Verification items for the finished model (mm, model axes). A direction names the side the tool comes from. Round coordinates to 2 decimals unless told otherwise and drop trailing zeros. Write each loop counter-clockwise with the first axis right and the second up, starting at its lowest first coordinate (ties: lowest second). Pieces come first, ordered by that corner, then holes. Notation, with made-up numbers: M 60,6 L 101,6 A16 ccw 101,23 Z; hole C -14.5,21.25 d7. An arc over 180 degrees is marked long. One line per item, written item: value. Start each with the question number.
from build123d import *

# Parameters (mm, degrees)
F0_R      = 146.05
F1_DEPTH  = 63.5
F2_R      = 142.875
F3_DEPTH  = 57.15
F5_DEPTH  = 57.15
F7_DEPTH  = 63.501
F8_W      = 381
F8_H      = 63.5
F9_DEPTH  = 6.35
F10_W     = 19.7993
F10_H     = 39.899997
F11_DEPTH = 6.35
F12_W     = 19.89836
F12_H     = 39.878
F13_DEPTH = 6.35
F14_R     = 50.8
F15_DEPTH = 6.35
F16_W     = 101.6
F16_H     = 81.28
F17_DEPTH = 63.501


with BuildPart() as f1:
    # F0 (on Top) → F1 (new body)
    with BuildSketch(Plane.XY):
        Circle(F0_R)
    extrude(amount=F1_DEPTH)

    # F2 (on face) → F3 (cut)
    with BuildSketch(Plane.XY.offset(63.5)):
        Circle(F2_R)
    extrude(amount=-F3_DEPTH, mode=Mode.SUBTRACT)

    # F4 (on face) → F5 (cut)
    with BuildSketch(Plane.XY.offset(63.5)):
        with BuildLine():
            Line((142.875, 0), (186.450183, 0))
            Line((186.450183, 0), (186.450183, 147.836223))
            Line((186.450183, 147.836223), (-190.863192, 147.836223))
            Line((-190.863192, 147.836223), (-190.863192, 0))
            Line((-190.863192, 0), (-142.875, 0))
            ThreePointArc((-142.875, 0), (0, 142.875), (142.875, 0))
        make_face()
    extrude(amount=-F5_DEPTH, mode=Mode.SUBTRACT)

    # F6 (on face) → F7 (cut, through all)
    with BuildSketch(Plane.XY.offset(63.5)):
        with BuildLine():
            Line((0, 0), (94.561977, 127.513117))
            ThreePointArc((94.561977, 127.513117), (0, 159.458628), (-94.561977, 127.513117))
            Line((-94.561977, 127.513117), (0, 0))
        make_face()
    extrude(amount=-F7_DEPTH, mode=Mode.SUBTRACT)

    # F8 (on Top) → F9 (join)
    with BuildSketch(Plane.XY):
        with Locations((0, 0.073786)):
            Rectangle(F8_W, F8_H)
    extrude(amount=F9_DEPTH)

    # F10 (on face) → F11 (cut)
    with BuildSketch(Plane.XY.offset(6.35)):
        with Locations((-159.01035, -0.826213)):
            Rectangle(F10_W, F10_H)
    extrude(amount=-F11_DEPTH, mode=Mode.SUBTRACT)

    # F12 (on Top) → F13 (cut)
    with BuildSketch(Plane.XY):
        with Locations((158.96082, -0.815214)):
            Rectangle(F12_W, F12_H)
    extrude(amount=F13_DEPTH, mode=Mode.SUBTRACT)

    # F14 (on Top) → F15 (cut)
    with BuildSketch(Plane.XY):
        Circle(F14_R)
    extrude(amount=F15_DEPTH, mode=Mode.SUBTRACT)

    # F16 (on Top) → F17 (cut, through all)
    with BuildSketch(Plane.XY):
        with Locations((0, 40.64)):
            Rectangle(F16_W, F16_H)
    extrude(amount=F17_DEPTH, mode=Mode.SUBTRACT)


solid = f1.part
1) Cross-section at B-B (z = 40). Record the boundary of the cut face in (x, y) (3 decimals).
2) Cross-section at A-A (x = -165). Record the boundary of the cut face in (y, z).
3) Access from +Z, -Z, +X, -X, +Y, -Y to the whole of each face (thin tool, end or side, straight path). Record for faces 4 (the cylindrical face through (-3.14, -142.84, 35.33)), 5 (the flat face through (-69.152, 93.249, 3.219)), 6 (the cylindrical face through (122.866, 78.959, 3.131)).
4) Gauge pin test, flat ends, axial feed: pin 1 Ø6 at (x, y) = (-57.5, 61.5) entering from +Z; pin 2 Ø5 at (y, z) = (44, 2) entering from +X; pin 3 Ø1 at (y, z) = (-35, 54) entering from +X. Record the tip position at first contact, or that the pin passes through.
5) Thickness scan on line 1 (Z direction, x = 71, y = 22); line 2 (X direction, y = -130, z = 39); line 3 (X direction, y = -35, z = 12). Record the ranges inside material, lowest first.
6) Cross-section at C-C (x = 0). Record the boundary of the cut face in (y, z) (3 decimals).
7) Mould release check, pull along X, two halves, no side actions. Record for faces 1 (the flat face through (-12, -143, 63.5)), 2 (the flat face through (68.65, 92.57, 3.22)), 3 (the cylindrical face through (-3.212, -146.015, 31.306)): pulls with the +X half, pulls with the -X half, needs draft (parallel to the pull), parting line crosses it, or undercut.
8) Cross-section at D-D (x = -65). Record the boundary of the cut face in (y, z), then the cut area to 3 significant figures.
Results below:
1. outline: M -146.05,0 A146.05 ccw 146.05,0 L 142.875,0 A142.875 cw -142.875,0 Z
2. outline: M -31.68,0 L -20.78,0 L -20.78,6.35 L -31.68,6.35 Z; M 19.12,0 L 31.82,0 L 31.82,6.35 L 19.12,6.35 Z
3. face 4: +Z, +Y
3. face 5: +Z, -Z, +Y
3. face 6: +Z, -Z, +X, +Y
4. pin 1: stops at z = 6.35
4. pin 2: stops at x = 140.03
4. pin 3: stops at x = 141.92
5. line 1: z = 0 to 6.35
5. line 2: x = -66.56 to -59.27, 59.27 to 66.56
5. line 3: x = -141.79 to -138.52, 138.52 to 141.79
6. outline: M -146.05,0 L -50.8,0 L -50.8,6.35 L -142.875,6.35 L -142.875,63.5 L -146.05,63.5 Z
7. face 1: needs draft
7. face 2: undercut
7. face 3: parting line crosses it
8. outline: M -130.79,0 L 87.65,0 L 87.65,6.35 L -127.23,6.35 L -127.23,63.5 L -130.79,63.5 Z
8. area: 1,590 mm²
